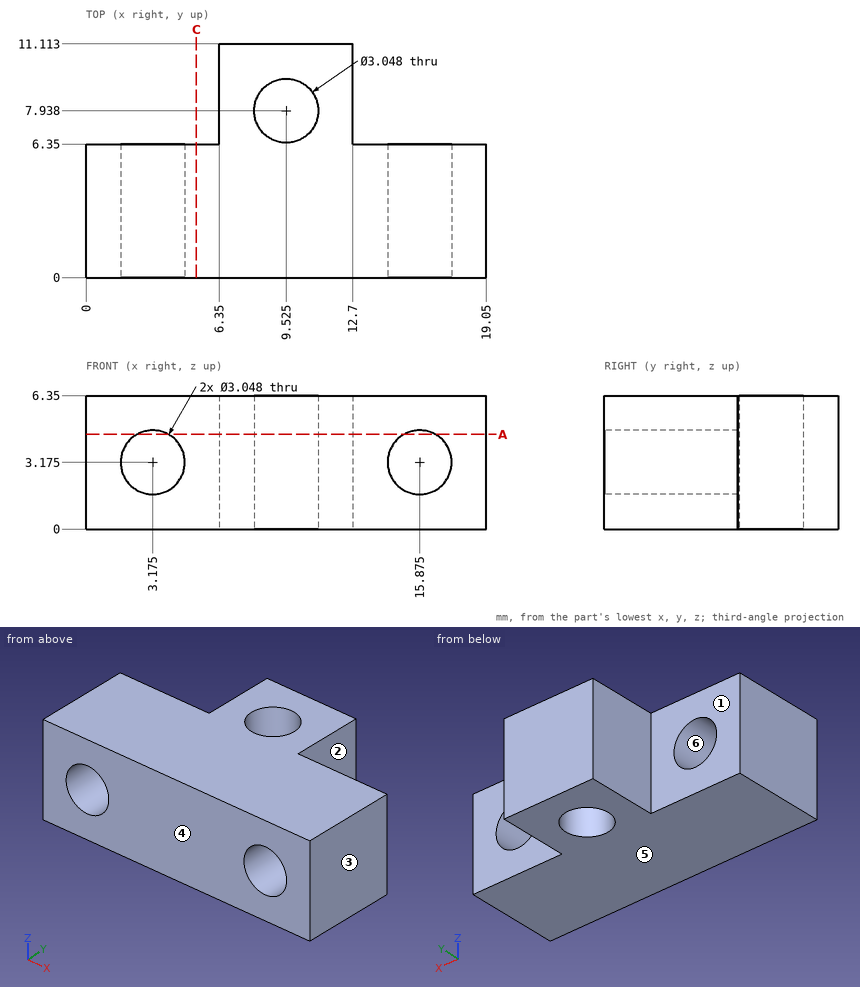
Input: dimensioned drawing with shaded views. Units: mm. Origin: part minimum x, y, z. A direction names the side the tool comes from. Coordinates: 2 decimals unless noted, no trailing zeros. Order: outer loops, then holes, each group sorted by start corner. A loop starts at its lowest first (then second) coordinate and runs counter-clockwise, first axis right, second up.
(1) Material intervals for probe 1 along Y at (x, z) = (9.5, 6); probe 2 along X at (y, z) = (2.75, 2.5); probe 3 along Y at (x, z) = (15.75, 6), sorted ascending.
(2) First-contact query: pin 1 (1.5 mm diameter, centred on x = 14.5, z = 3, fed in from +Y); pin 2 (2.5 mm diameter, centred on x = 15.875, z = 3.175, fed in from +Y); pin 3 (2.5 mm diameter, centred on y = 8.5, z = 2, fed in from -X). Flat tips, straight axial feed; report the tip coordinate or a pass-through.
(3) Draft query along Z for the marked faces 4, 5 and 6. Return one class per face: pulls with the +Z half, pulls with the -Z half, needs draft (parallel to the pull), parting line crosses it, or undercut.
(4) Access query for the marked faces 1, 2 and 3. Directions: +Z, -Z, +X, -X, +Y, -Y. A direction counts if a zero-diameter tool reaches every point of the face in a straight line with its end or side. Return the directions, or none.
(5) Section query A-A (z = 4.5). State how many separate pieces and enclosed holes the cut face has, plus the area to 3 significant figures.
(6) Section query C-C (x = 5.25). Return the cut outline in (y, z), plus the area to 3 significant figures.
Solution:
1. probe 1: y = 0 to 6.41, 9.46 to 11.11
1. probe 2: x = 0 to 1.81, 4.54 to 14.51, 17.24 to 19.05
1. probe 3: y = 0 to 6.35
2. pin 1: stops at y = 6.35
2. pin 2: passes through
2. pin 3: stops at x = 6.35
3. face 4: needs draft
3. face 5: pulls with the -Z half
3. face 6: undercut
4. face 1: +Z, -Z, -X, +Y
4. face 2: +Z, -Z, +X, +Y
4. face 3: +Z, -Z, +X, +Y, -Y
5. separate pieces: 3
5. enclosed holes: 1
5. area: 125 mm2
6. outline: (0, 0) - (6.35, 0) - (6.35, 6.35) - (0, 6.35) - close
6. area: 40.3 mm2
